Part model, mm, in its own coordinate system. A direction names the side the tool comes from. Round coordinates to 2 decimals unless told otherwise and drop trailing zeros. Loops run counter-clockwise (first coordinate to the right, second up) from the corner with the lowest first, then second, coordinate; pieces in that order, holes last.
from build123d import *

# Parameters (mm, degrees)
F0_R     = 2.5
F1_DEPTH = 3
F2_DEPTH = 10


with BuildPart() as f1:
    # F0 (on Top) → F1 (new body)
    with BuildSketch(Plane.XY):
        with BuildLine():
            ThreePointArc((0, 4), (1.171573, 1.171573), (4, 0))
            Line((4, 0), (66, 0))
            ThreePointArc((66, 0), (68.828427, 1.171573), (70, 4))
            Line((70, 4), (70, 66))
            ThreePointArc((70, 66), (68.828427, 68.828427), (66, 70))
            Line((66, 70), (4, 70))
            ThreePointArc((4, 70), (1.171573, 68.828427), (0, 66))
            Line((0, 66), (0, 4))
        make_face()
        with Locations((5, 5)):
            Circle(F0_R, mode=Mode.SUBTRACT)
        with Locations((65, 5)):
            Circle(F0_R, mode=Mode.SUBTRACT)
        with Locations((5, 65)):
            Circle(F0_R, mode=Mode.SUBTRACT)
        Polygon((45, 25), (42.5, 25), (27.5, 25), (25, 25), (25, 47.5), (45, 47.5), align=None, mode=Mode.SUBTRACT)
        with Locations((65, 65)):
            Circle(F0_R, mode=Mode.SUBTRACT)
    extrude(amount=F1_DEPTH)

    # F0 (on Top) → F2 (join)
    with BuildSketch(Plane.XY):
        Polygon((42.5, 45), (42.5, 25), (45, 25), (45, 47.5), (25, 47.5), (25, 25), (27.5, 25), (27.5, 45), align=None)
    extrude(amount=F2_DEPTH)


solid = f1.part
1) Mould opens along X. For faces 5 (the face through (1.141, 1.203, 1.479)), 6 (the face through (68.797, 1.141, 1.479)), 7 (the face through (67.385, 5.751, 1.479)), 8 (the face through (35, 0, 1)) say: released by +X, released by -X, zero draft, split by the parting line, or undercut.
Values:
face 5: released by -X
face 6: released by +X
face 7: undercut
face 8: zero draft
2) Wall check: line 1 along Y through (x, z) = (65, 0.8); line 2 along Y through (x, z) = (37.5, 2.5); line 3 along X through (y, z) = (42, 1.75). Give the ranges that are in metal, low to high.
Values:
line 1: y = 0 to 2.5, 7.5 to 62.5, 67.5 to 70
line 2: y = 0 to 25, 45 to 70
line 3: x = 0 to 27.5, 42.5 to 70
3) Slice it at D-D, the plane z = 1.5. Give the cut face in (x, y), then the cut area to 3 significant figures.
Values:
outline: (0, 4) arc R4 ccw to (4, 0) - (66, 0) arc R4 ccw to (70, 4) - (70, 66) arc R4 ccw to (66, 70) - (4, 70) arc R4 ccw to (0, 66) - close; hole circle Ø5 at (5, 5); hole circle Ø5 at (5, 65); hole (27.5, 25) - (42.5, 25) - (42.5, 45) - (27.5, 45) - close; hole circle Ø5 at (65, 5); hole circle Ø5 at (65, 65)
area: 4,510 mm2
4) Slice it at A-A, the plane x = 5. Give the cut face in (y, z).
Values:
outline: (0, 0) - (2.5, 0) - (2.5, 3) - (0, 3) - close; (7.5, 0) - (62.5, 0) - (62.5, 3) - (7.5, 3) - close; (67.5, 0) - (70, 0) - (70, 3) - (67.5, 3) - close
5) Slice it at C-C, the plane x = 41. Give the cut face in (y, z).
Values:
outline: (0, 0) - (25, 0) - (25, 3) - (0, 3) - close; (45, 0) - (70, 0) - (70, 3) - (47.5, 3) - (47.5, 10) - (45, 10) - close
6) Drop flat-ended pins along their axis: pin 1 Ø2 at (x, z) = (26, 5.5) entering from -Y; pin 2 Ø6.5 at (x, y) = (65, 65) entering from +Z; pin 3 Ø2 at (y, z) = (34, 8) entering from +X. Give the stop position or say it passes through.
Values:
pin 1: stops at y = 25
pin 2: stops at z = 3
pin 3: stops at x = 45
7) Tool access for faces 1 (the face through (42.5, 35, 5)), 2 (the face through (1.203, 68.859, 1.479)), 3 (the face through (26, 25, 6)), 4 (the face through (35, 47.5, 6)): list every direction of +Z, -Z, +X, -X, +Y, -Y with a clear straight run to the whole face (end or side of a thin tool).
Values:
face 1: +Z, -Z
face 2: +Z, -Z, -X, +Y
face 3: +Z, +X, -X, -Y
face 4: +Z, +X, -X, +Y
